Geometry check sheet. Reference: the model listing, model coordinates, mm. Face numbers are marked on the shaded views. A direction names the side the tool comes from. Give positions to 0.01 mm unless a question says otherwise; leave off trailing zeros. Loops run counter-clockwise (first coordinate to the right, second up) from the corner with the lowest first, then second, coordinate; pieces in that order, holes last. Notation, with made-up numbers: (52.25, -1.5) -> (101.25, -1.5) arc R26 ccw to (101.25, 14.5) -> close; hole circle Ø6 at (-6.75, 80). An arc over 180 degrees is marked (long way). Write item = value, one per line.
```python
from build123d import *

# Parameters (mm, degrees)
BOSS_EXTRUDE1_DEPTH = 6
BOSS_EXTRUDE2_DEPTH = 2.5
BOSS_EXTRUDE3_DEPTH = 3.5
BOSS_EXTRUDE4_DEPTH = 4


with BuildPart() as part:
    # Sketch1 → Boss-Extrude1 (new, symmetric)
    with BuildSketch(Plane(origin=(0, 0, 0), x_dir=(1, 0, 0), z_dir=(0, 1, 0))):
        with BuildLine():
            ThreePointArc((8.92789337, 3.662679343), (0, 9.65), (-8.92789337, 3.662679343))
            add(Edge.make_bspline(
                [(-8.724914389, 6.107239058), (-8.904858788, 5.893861034), (-9.803458989, 4.322571827), (-8.92789337, 3.662679343)],
                knots=[0, 0, 0, 0, 1, 1, 1, 1], degree=3))
            ThreePointArc((-8.724914389, 6.107239058), (0, 10.65), (8.724914389, 6.107239058))
            add(Edge.make_bspline(
                [(8.724914389, 6.107239058), (8.904858788, 5.893861034), (9.803458989, 4.322571827), (8.92789337, 3.662679343)],
                knots=[0, 0, 0, 0, 1, 1, 1, 1], degree=3))
        make_face()
    extrude(amount=BOSS_EXTRUDE1_DEPTH, both=True)

    # Sketch2 → Boss-Extrude2 (add, symmetric)
    with BuildSketch(Plane(origin=(0, 0, 0), x_dir=(1, 0, 0), z_dir=(0, 1, 0))):
        with BuildLine():
            Line((-7.75, 13.180055627), (-7.75, 6.976773921))
            Line((-7.75, 6.976773921), (-7, 6.976773921))
            Line((-7, 6.976773921), (-7, 13.180055627))
            ThreePointArc((-7, 13.180055627), (0, 20.180055627), (7, 13.180055627))
            Line((7, 13.180055627), (7, 6.976773921))
            Line((7, 6.976773921), (7.75, 6.976773921))
            Line((7.75, 6.976773921), (7.75, 13.180055627))
            ThreePointArc((7.75, 13.180055627), (0, 20.930055627), (-7.75, 13.180055627))
        make_face()
    extrude(amount=BOSS_EXTRUDE2_DEPTH, both=True)

    # Sketch3 → Boss-Extrude3 (add, symmetric)
    with BuildSketch(Plane(origin=(0, 0, 0), x_dir=(1, 0, 0), z_dir=(0, 1, 0))):
        with BuildLine():
            add(Edge.make_bspline(
                [(-7.25611922, 9.254992682), (-7.041583851, 11.20624294), (-5.98153876, 11.097373504), (-5.637887905, 10.914088424)],
                knots=[0, 0, 0, 0, 1, 1, 1, 1], degree=3))
            Line((-5.637887905, 10.914088424), (-4.051396134, 9.849298928))
            ThreePointArc((-4.051396134, 9.849298928), (-5.858619381, 8.893766297), (-7.449979396, 7.610539205))
            Line((-7.449979396, 7.610539205), (-7.25611922, 9.254992682))
        make_face()
        with BuildLine():
            Line((7.449979396, 7.610539205), (7.25611922, 9.254992682))
            add(Edge.make_bspline(
                [(7.25611922, 9.254992682), (7.041583851, 11.20624294), (5.98153876, 11.097373504), (5.637887905, 10.914088424)],
                knots=[0, 0, 0, 0, 1, 1, 1, 1], degree=3))
            Line((5.637887905, 10.914088424), (4.051396134, 9.849298928))
            ThreePointArc((4.051396134, 9.849298928), (5.858619381, 8.893766297), (7.449979396, 7.610539205))
        make_face()
    extrude(amount=BOSS_EXTRUDE3_DEPTH, both=True)

    # Sketch4 → Boss-Extrude4 (add, symmetric)
    with BuildSketch(Plane(origin=(0, 0, 0), x_dir=(1, 0, 0), z_dir=(0, 1, 0))):
        with BuildLine():
            ThreePointArc((6.013295106, 7.547369208), (0, 9.65), (-6.013295106, 7.547369208))
            add(Edge.make_bspline(
                [(-5.359344629, 7.661587639), (-5.783257591, 7.437743582), (-6.013295106, 7.547369208)],
                knots=[0, 0, 0, 1, 1, 1], degree=2))
            ThreePointArc((-5.359344629, 7.661587639), (0, 9.35), (5.359344629, 7.661587639))
            add(Edge.make_bspline(
                [(5.359344629, 7.661587639), (5.783257591, 7.437743582), (6.013295106, 7.547369208)],
                knots=[0, 0, 0, 1, 1, 1], degree=2))
        make_face()
    extrude(amount=BOSS_EXTRUDE4_DEPTH, both=True)


solid = part.part
```
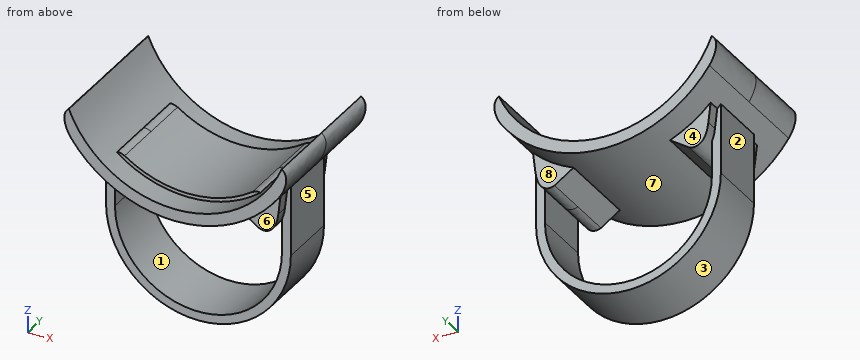
Item 1: Section check A-A, the plane z = -12.25. Record the cut outline in (x, y).
Answer:
outline = (-7.75, -2.5) -> (-7, -2.5) -> (-7, 2.5) -> (-7.75, 2.5) -> close; (7, -2.5) -> (7.75, -2.5) -> (7.75, 2.5) -> (7, 2.5) -> close
Item 2: Section check D-D, the plane x = 2. Record the cut outline in (y, z).
Answer:
outline = (-6, -10.46) -> (6, -10.46) -> (6, -9.44) -> (4, -9.44) -> (4, -9.13) -> (-4, -9.13) -> (-4, -9.44) -> (-6, -9.44) -> close; (-2.5, -20.67) -> (2.5, -20.67) -> (2.5, -19.89) -> (-2.5, -19.89) -> close
Item 3: Section check C-C, the plane z = -6.75. Record the cut outline in (x, y), plus the area to 3 significant figures.
Answer:
outline = (-8.24, -6) -> (-6.9, -6) -> (-6.9, 6) -> (-8.24, 6) -> close; (6.9, -6) -> (8.24, -6) -> (8.24, 6) -> (6.9, 6) -> close
area = 32.2 mm^2
Item 4: Thickness scan on L1, parallel to X at y = -2.25, z = -12.5; L2, parallel to Z at x = -4.25, y = -2.25; L3, parallel to Z at x = 2.25, y = 1. Record the ranges inside material, lowest first. Write a range as [from, to].
Answer:
L1 = [-7.75, -7], [7, 7.75]
L2 = [-19.66, -18.74], [-9.98, -8.33]
L3 = [-20.6, -19.81], [-10.41, -9.08]
Item 5: Tool access check on the marked faces 4, 5, 6, 7 and 8. Record the directions out of +Z, -Z, +X, -X, +Y, -Y that give a thin tool (end or side, any length) a straight path to the whole face; none if there is none.
Answer:
face_4 = -Z, -X, +Y
face_5 = -Z, +X, +Y, -Y
face_6 = -Z, +X, -Y
face_7 = none
face_8 = -Z, +X, +Y
Item 6: Gauge pin test, flat ends, axial feed: pin 1 (2 mm diameter, centred on x = -7.5, z = -15, fed in from -Y); pin 2 (2 mm diameter, centred on y = 0.5, z = -7, fed in from +X); pin 3 (2 mm diameter, centred on x = -5.5, y = 2, fed in from -Z). Record the tip position at first contact, or that the pin passes through.
Answer:
pin_1 = -2.5
pin_2 = 8.8
pin_3 = -19.49
Item 7: Draft check along X on the marked faces 1, 2 and 3. Enter one of: +X half, -X half, draft (parallel to the pull), parting line (faces both ways), or undercut.
Answer:
face_1 = undercut
face_2 = -X half
face_3 = parting line
Item 8: Section check B-B, the plane x = 0. Record the cut outline in (y, z).
Answer:
outline = (-6, -10.65) -> (6, -10.65) -> (6, -9.65) -> (4, -9.65) -> (4, -9.35) -> (-4, -9.35) -> (-4, -9.65) -> (-6, -9.65) -> close; (-2.5, -20.93) -> (2.5, -20.93) -> (2.5, -20.18) -> (-2.5, -20.18) -> close
